from build123d import *

# Parameters (mm, degrees)
SKETCH2_R          = 1.6
CUT_EXTRUDE1_DEPTH = 10


with BuildPart() as part:
    # Sketch1 → Revolve1 (revolve)
    with BuildSketch(Plane.XY, mode=Mode.PRIVATE) as revolve1_sk:
        Polygon((0, -2.5), (0, -6), (7, -6), (7, -4), (17, -4), (17, -6), (24, -6), (24, -2.5), align=None)
    revolve(revolve1_sk.sketch.rotate(Axis((0, 0, 0), (1, 0, 0)), 270), axis=Axis((0, 0, 0), (1, 0, 0)))

    # Sketch2 → Cut-Extrude1 (cut)
    with BuildSketch(Plane(origin=(0, 0, 0), x_dir=(1, 0, 0), z_dir=(0, 1, 0))):
        with Locations(Location((3.5, 0, 0), (0, 0, 90))):
            Circle(SKETCH2_R)
        with Locations(Location((20.5, 0, 0), (0, 0, 90))):
            Circle(SKETCH2_R)
    extrude(amount=CUT_EXTRUDE1_DEPTH, mode=Mode.SUBTRACT)


solid = part.part
Model file for the job. Use its own axes, mm. A direction names the side the tool comes from. Give positions to 0.01 mm unless a question says otherwise; leave off trailing zeros. Loops run counter-clockwise (first coordinate to the right, second up) from the corner with the lowest first, then second, coordinate; pieces in that order, holes last.
1) Tool access for faces 1 (the cylindrical face through (12.07, 3.905, -0.867)), 2 (the cylindrical face through (20.549, -5.059, 3.226)), 3 (the cylindrical face through (3.019, 3.935, -1.526)): list every direction of +Z, -Z, +X, -X, +Y, -Y with a clear straight run to the whole face (end or side of a thin tool).
2) Saw through at C-C (y = 5). Write the cut outline in (x, z), plus the area to 3 significant figures.
3) Saw through at A-A (z = 0). Write the cut outline in (x, y).
4) Pull direction X, two halves, no side cores. Call faces 4 (the flat face through (24, 0, 3)), 5 (the cylindrical face through (20.019, 3.935, -1.526)), 6 (the flat face through (0, 0, -3)): +X half, -X half, draft (parallel to the pull), parting line (faces both ways), or undercut.
5) Saw through at D-D (z = -5). Write the cut outline in (x, y), plus the area to 3 significant figures.
6) Saw through at B-B (y = 1). Write the cut outline in (x, z), plus the area to 3 significant figures.
7) Wall check: line 1 (X direction, y = 3.75, z = 0); line 2 (X direction, y = -3.75, z = -4.25); line 3 (X direction, y = 4.05, z = 0). Give the ranges that are in metal, low to high.
8) Flat gauge pins, fed straight in: pin 1 Ø4 at (x, z) = (17.5, -4.5) entering from -Y; pin 2 Ø3 at (y, z) = (0, 0) entering from +X; pin 3 Ø1.5 at (x, y) = (9.5, -1.5) entering from +Z; pin 4 Ø4 at (x, z) = (6.5, 3.5) entering from +Y. Where does each tip first touch, or does it go through?
Answer block:
1. face 1: none
1. face 2: +X, -X
1. face 3: +Y
2. outline: (0, -3.32) - (7, -3.32) - (7, 3.32) - (0, 3.32) - close; (17, -3.32) - (24, -3.32) - (24, 3.32) - (17, 3.32) - close; hole circle Ø3.2 at (3.5, 0); hole circle Ø3.2 at (20.5, 0)
2. area: 76.8 mm2
3. outline: (0, -6) - (7, -6) - (7, -4) - (17, -4) - (17, -6) - (24, -6) - (24, -2.5) - (0, -2.5) - close; (0, 2.5) - (1.9, 2.5) - (1.9, 6) - (0, 6) - close; (5.1, 2.5) - (18.9, 2.5) - (18.9, 6) - (17, 6) - (17, 4) - (7, 4) - (7, 6) - (5.1, 6) - close; (22.1, 2.5) - (24, 2.5) - (24, 6) - (22.1, 6) - close
4. face 4: +X half
4. face 5: undercut
4. face 6: -X half
5. outline: (0, -3.32) - (7, -3.32) - (7, 3.32) - (0, 3.32) - close; (17, -3.32) - (24, -3.32) - (24, 3.32) - (17, 3.32) - close
5. area: 92.9 mm2
6. outline: (0, -5.92) - (7, -5.92) - (7, -3.87) - (17, -3.87) - (17, -5.92) - (24, -5.92) - (24, -2.29) - (0, -2.29) - close; (0, 2.29) - (24, 2.29) - (24, 5.92) - (17, 5.92) - (17, 3.87) - (7, 3.87) - (7, 5.92) - (0, 5.92) - close
6. area: 133 mm2
7. line 1: x = 0 to 1.9, 5.1 to 18.9, 22.1 to 24
7. line 2: x = 0 to 7, 17 to 24
7. line 3: x = 0 to 1.9, 5.1 to 7, 17 to 18.9, 22.1 to 24
8. pin 1: stops at y = -5.45
8. pin 2: passes through
8. pin 3: stops at z = 3.93
8. pin 4: stops at y = 5.81
